Design review of the part built by this model. Coordinates are the model's own, in mm. Face numbers are marked on the shaded views. A direction names the side the tool comes from. Give positions to 0.01 mm unless a question says otherwise; leave off trailing zeros. Loops run counter-clockwise (first coordinate to the right, second up) from the corner with the lowest first, then second, coordinate; pieces in that order, holes last. Notation, with made-up numbers: (25.5, -5.5) -> (65.5, -5.5) arc R23 cw to (65.5, 11.5) -> close; hole circle Ø7 at (-14.75, 86). An arc over 180 degrees is marked (long way). Use a Markdown table: item, result. Add a question column.
1. For pin 1 Ø1.6 at (x, z) = (41, 20.5) entering from -Y; pin 2 Ø1.6 at (y, z) = (37, 10) entering from -X; pin 3 Ø2 at (x, z) = (41.5, 20) entering from +Y; pin 4 Ø1.6 at (x, y) = (17, 34) entering from -Z, all flat-tipped, find the tip position at first contact; note any pin that passes through.
2. To check wall thickness, follow line 1 (Y direction, x = 3.5, z = 15.25); line 2 (Z direction, x = 40.7, y = 24.5); line 3 (X direction, y = 1, z = 11). State the ranges of each line that lie inside material, in increasing order.
3. Add section C-C (x = -28.5). State the section outline as (y, z) points.
4. For the marked faces 1 and 2, list the 3-axis set-ups (+Z, -Z, +X, -X, +Y, -Y) from which the entire face can be reached by the end or side of a thin tool; tool diameter is ignored.
5. Add section D-D (y = -31.5). State the section outline as (x, z) points.
6. Add section B-B (z = 3.5). State the section outline as (x, y) points, and give its area (3 significant figures).
7. Add section A-A (y = 4). State the section outline as (x, z) points, and give its area (3 significant figures).
```python
from build123d import *

# Parameters (mm, degrees)
F0_W     = 80
F0_H     = 71
F1_DEPTH = 2
F0_W_2   = 84
F0_H_2   = 75
F2_DEPTH = 30
F3_R     = 4
F4_DEPTH = 25
F5_W     = 18
F5_H     = 6
F6_DEPTH = 25
F5_W_2   = 17.5
F5_H_2   = 12.5
F5_W_3   = 13.5
F5_H_3   = 8.5
F7_DEPTH = 2
F5_R     = 3.25
F8_DEPTH = 25
F3_W     = 2
F3_H     = 3.5
F9_DEPTH = 25
F10_R    = 3
F11_R    = 3


with BuildPart() as f1:
    # F0 (on Top) → F1 (new body)
    with BuildSketch(Plane.XY):
        Rectangle(F0_W, F0_H)
    extrude(amount=F1_DEPTH)

    # F0 (on Top) → F2 (join)
    with BuildSketch(Plane.XY):
        Rectangle(F0_W_2, F0_H_2)
        Rectangle(F0_W, F0_H, mode=Mode.SUBTRACT)
    extrude(amount=F2_DEPTH)

    # F3 (on face) → F4 (cut)
    with BuildSketch(Plane(origin=(40, 0, 0), x_dir=(0, -1, 0), z_dir=(-1, 0, 0))):
        with Locations((-24.5, 20)):
            Circle(F3_R)
        with Locations((-4, 20)):
            Circle(F3_R)
        with Locations((16.5, 20)):
            Circle(F3_R)
    extrude(amount=-F4_DEPTH, mode=Mode.SUBTRACT)

    # F5 (on face) → F6 (cut)
    with BuildSketch(Plane.XZ.offset(-35.5)):
        with Locations((-9, 9)):
            Rectangle(F5_W, F5_H)
    extrude(amount=-F6_DEPTH, mode=Mode.SUBTRACT)

    # F5 (on face) → F7 (join)
    with BuildSketch(Plane.XZ.offset(-35.5)):
        with Locations((20, 20)):
            Rectangle(F5_W_2, F5_H_2)
        with Locations((20, 20)):
            Rectangle(F5_W_3, F5_H_3, mode=Mode.SUBTRACT)
    extrude(amount=F7_DEPTH)

    # F5 (on face) → F8 (cut)
    with BuildSketch(Plane.XZ.offset(-35.5)):
        with Locations((20, 20)):
            Circle(F5_R)
    extrude(amount=-F8_DEPTH, mode=Mode.SUBTRACT)

    # F3 (on face) → F9 (cut)
    with BuildSketch(Plane(origin=(40, 0, 0), x_dir=(0, -1, 0), z_dir=(-1, 0, 0))):
        with Locations((-16.5, 20)):
            Rectangle(F3_W, F3_H)
        with Locations((4, 20)):
            Rectangle(F3_W, F3_H)
        with Locations((24.5, 20)):
            Rectangle(F3_W, F3_H)
    extrude(amount=-F9_DEPTH, mode=Mode.SUBTRACT)

    # F10
    f10_edges = [f1.edges().sort_by_distance(p)[0] for p in [
        (40, 35.5, 16),
        (-40, 35.5, 16),
        (-40, -35.5, 16),
        (40, -35.5, 16),
    ]]
    fillet(f10_edges, radius=F10_R)

    # F11
    f11_edges = [f1.edges().sort_by_distance(p)[0] for p in [
        (42, -37.5, 15),
        (42, 37.5, 15),
        (-42, -37.5, 15),
        (-42, 37.5, 15),
    ]]
    fillet(f11_edges, radius=F11_R)


solid = f1.part
```
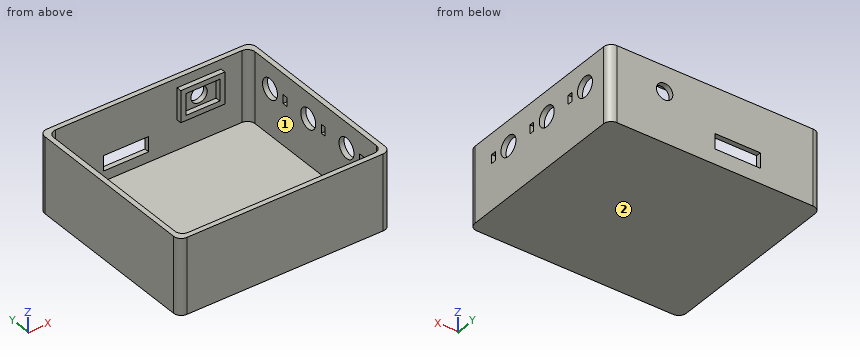
Taken from the geometry:
| question | item | result |
|---|---|---|
| 1 | pin 1 | stops at y = -37.25 |
| 1 | pin 2 | stops at x = -41.47 |
| 1 | pin 3 | stops at y = 37.1 |
| 1 | pin 4 | stops at z = 0 |
| 2 | line 1 | y = -37.5 to -35.5, 35.5 to 37.5 |
| 2 | line 2 | z = 0 to 16, 24 to 30 |
| 2 | line 3 | x = -42 to -40, 40 to 42 |
| 3 | outline | (-37.5, 0) -> (37.5, 0) -> (37.5, 30) -> (35.5, 30) -> (35.5, 2) -> (-35.5, 2) -> (-35.5, 30) -> (-37.5, 30) -> close |
| 4 | face 1 | +Z |
| 4 | face 2 | -Z, +X, -X, +Y, -Y |
| 5 | outline | (-42, 0) -> (42, 0) -> (42, 30) -> (40, 30) -> (40, 2) -> (-40, 2) -> (-40, 30) -> (-42, 30) -> close |
| 6 | outline | (-42, -34.5) arc R3 ccw to (-39, -37.5) -> (39, -37.5) arc R3 ccw to (42, -34.5) -> (42, 34.5) arc R3 ccw to (39, 37.5) -> (-39, 37.5) arc R3 ccw to (-42, 34.5) -> close; hole (-40, -32.5) arc R3 ccw to (-37, -35.5) -> (37, -35.5) arc R3 ccw to (40, -32.5) -> (40, 32.5) arc R3 ccw to (37, 35.5) -> (-37, 35.5) arc R3 ccw to (-40, 32.5) -> close |
| 6 | area | 620 mm^2 |
| 7 | outline | (-42, 0) -> (42, 0) -> (42, 16) -> (40, 16) -> (40, 2) -> (-40, 2) -> (-40, 30) -> (-42, 30) -> close; (40, 24) -> (42, 24) -> (42, 30) -> (40, 30) -> close |
| 7 | area | 264 mm^2 |
